Can you work these out from the model? Positions are in its coordinate system, mm. Face numbers are marked on the shaded views. A direction names the side the tool comes from. Coordinates: 2 decimals unless noted, no trailing zeros. Order: outer loops, then holes, each group sorted by start corner. A loop starts at its lowest first (then second) coordinate and runs counter-clockwise, first axis right, second up. Notation, with made-up numbers: (89, -7.5) -> (103, -7.5) arc R15 ccw to (103, -3.5) -> close; hole circle Ø2 at (69, 55.25). An arc over 180 degrees is marked (long way). Answer as a JSON object with one key per item and string values. Group by question number.
(1) If we mould it in two halves opening along Y, with no side actions, what happens to the marked faces 1, 2 and 3? For each: pulls with the +Y half, pulls with the -Y half, needs draft (parallel to the pull), parting line crosses it, or undercut.
(2) I need wall thicknesses on line 1 (Y direction, x = 0, z = 6.8); line 2 (Y direction, x = 0, z = 2.2); line 3 (Z direction, x = -1.5, y = -4). Which ranges of each line are inside material? Lowest first, please.
(3) I want a section at D-D, the plane z = 1.25. List the corners of the cut face in (x, y) for me.
(4) Which directions (+Z, -Z, +X, -X, +Y, -Y) give clear straight access to the entire face, cutting with the end or side of a thin tool? Please do the marked faces 4, 5 and 6.
(5) For pin 1 (5 mm diameter, centred on x = 3, z = 3.5, fed in from -Y); pin 2 (1.8 mm diameter, centred on x = 1, y = 0, fed in from +Z); pin 3 (3 mm diameter, centred on x = 3, z = 6, fed in from -Y), each with a flat end and sliding along its axis, tell me the tip position at first contact or that it passes through.
(6) I want a section at A-A, the plane y = 0. List the corners of the cut face in (x, z) for me.
(7) I want a section at C-C, the plane z = 6.5. List the corners of the cut face in (x, y) for me, plus the area to 3 significant figures.
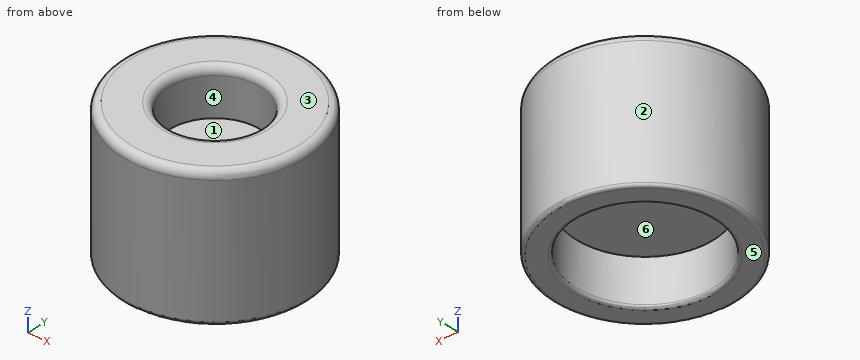
from build123d import *

# Parameters (mm, degrees)
SKETCH_1_R          = 6
SKETCH_1_R_2        = 4.5
EXTRUDE_1_DEPTH     = 3
SKETCH_2_R          = 6
EXTRUDE_2_DEPTH     = 6
SKETCH_3_R          = 3
CUT_EXTRUDE_1_DEPTH = 3
FILLET_1_R          = 0.5
FILLET_2_R          = 0.5
FILLET_3_R          = 0.2


with BuildPart() as part:
    # 草图1 → 凸台-拉伸1 (new body)
    with BuildSketch(Plane.XY):
        Circle(SKETCH_1_R)
        Circle(SKETCH_1_R_2, mode=Mode.SUBTRACT)
    extrude(amount=EXTRUDE_1_DEPTH)

    # 草图2 → 凸台-拉伸2 (add)
    with BuildSketch(Plane.XY.offset(3)):
        Circle(SKETCH_2_R)
    extrude(amount=EXTRUDE_2_DEPTH)

    # 草图3 → 切除-拉伸1 (cut)
    with BuildSketch(Plane.XY.offset(9)):
        Circle(SKETCH_3_R)
    extrude(amount=-CUT_EXTRUDE_1_DEPTH, mode=Mode.SUBTRACT)

    # 圆角1
    fillet_1_edges = [part.edges().sort_by_distance(p)[0] for p in [
        (-3, 0, 9),
    ]]
    fillet(fillet_1_edges, radius=FILLET_1_R)

    # 圆角2
    fillet_2_edges = [part.edges().sort_by_distance(p)[0] for p in [
        (-6, 0, 9),
    ]]
    fillet(fillet_2_edges, radius=FILLET_2_R)

    # 圆角3
    fillet_3_edges = [part.edges().sort_by_distance(p)[0] for p in [
        (-6, 0, 0),
        (-4.5, 0, 0),
    ]]
    fillet(fillet_3_edges, radius=FILLET_3_R)


solid = part.part
Computed values:
{
 "1": {"face 1": "undercut", "face 2": "parting line crosses it", "face 3": "needs draft"},
 "2": {"line 1": "y = -6 to -3, 3 to 6", "line 2": "y = -6 to -4.5, 4.5 to 6", "line 3": "z = 3 to 9"},
 "3": {"outline": "circle Ø12 at (0, 0); hole circle Ø9 at (0, 0)"},
 "4": {"face 4": "+Z", "face 5": "-Z, +X, -X, +Y, -Y", "face 6": "-Z"},
 "5": {"pin 1": "stops at y = -5.98", "pin 2": "stops at z = 6", "pin 3": "stops at y = -5.81"},
 "6": {"outline": "(-6, 0.2) arc R0.2 ccw to (-5.8, 0) -> (-4.7, 0) arc R0.2 ccw to (-4.5, 0.2) -> (-4.5, 3) -> (4.5, 3) -> (4.5, 0.2) arc R0.2 ccw to (4.7, 0) -> (5.8, 0) arc R0.2 ccw to (6, 0.2) -> (6, 8.5) arc R0.5 ccw to (5.5, 9) -> (3.5, 9) arc R0.5 ccw to (3, 8.5) -> (3, 6) -> (-3, 6) -> (-3, 8.5) arc R0.5 ccw to (-3.5, 9) -> (-5.5, 9) arc R0.5 ccw to (-6, 8.5) -> close"},
 "7": {"outline": "circle Ø12 at (0, 0); hole circle Ø6 at (0, 0)", "area": "84.8 mm2"}
}
